Input: part model. Units: mm. Frame: model coordinates. A direction names the side the tool comes from. Give positions to 0.01 mm unless a question says otherwise; leave off trailing zeros. Write each loop counter-clockwise with the first axis right and the second up, starting at its lowest first coordinate (ties: lowest second). Pieces come first, ordered by that corner, then holes.
```python
from build123d import *

# Parameters (mm, degrees)
SKETCH1_W           = 85
SKETCH1_H           = 52.5
BOSS_EXTRUDE1_DEPTH = 27
SKETCH2_R           = 2.5
CUT_EXTRUDE1_DEPTH  = 104.490337713
SKETCH4_W           = 24.5
SKETCH4_H           = 12.7
CUT_EXTRUDE2_DEPTH  = 104.490337713
SKETCH5_W           = 25
SKETCH5_H           = 12.7
CUT_EXTRUDE3_DEPTH  = 94.477269964
SKETCH6_W           = 40.9
SKETCH6_H           = 28
CUT_EXTRUDE4_DEPTH  = 104.490337713
FILLET1_R           = 10
FILLET2_R           = 8
FILLET4_R           = 2
SKETCH7_R           = 2.75
CUT_EXTRUDE5_DEPTH  = 104.490337713
SKETCH8_W           = 6
SKETCH8_H           = 1.5
CUT_EXTRUDE6_DEPTH  = 2
CUT_EXTRUDE7_DEPTH  = 101.924427172
BOSS_EXTRUDE2_START = 17
BOSS_EXTRUDE2_DEPTH = 17
SKETCH11_R          = 2.75
CUT_EXTRUDE8_DEPTH  = 104.490337713
FILLET5_R           = 2


with BuildPart() as part:
    # Sketch1 → Boss-Extrude1 (new body)
    with BuildSketch(Plane(origin=(0, 0, 0), x_dir=(1, 0, 0), z_dir=(0, 1, 0))):
        with Locations((42.5, 26.25)):
            Rectangle(SKETCH1_W, SKETCH1_H)
    extrude(amount=BOSS_EXTRUDE1_DEPTH)

    # Sketch2 → Cut-Extrude1 (cut, through all)
    with BuildSketch(Plane(origin=(0, 27, 0), x_dir=(1, 0, 0), z_dir=(0, 1, 0))):
        with Locations(Location((5.5, 41.5, 0), (0, 0, 270))):
            Circle(SKETCH2_R)
        with Locations(Location((53.5, 41.5, 0), (0, 0, 270))):
            Circle(SKETCH2_R)
        with Locations(Location((53.5, 33.7, 0), (0, 0, 270))):
            Circle(SKETCH2_R)
        with Locations(Location((5.5, 33.7, 0), (0, 0, 270))):
            Circle(SKETCH2_R)
    extrude(amount=-CUT_EXTRUDE1_DEPTH, mode=Mode.SUBTRACT)

    # Sketch4 → Cut-Extrude2 (cut, through all)
    with BuildSketch(Plane.ZY):
        with Locations((-12.25, 20.65)):
            Rectangle(SKETCH4_W, SKETCH4_H)
    extrude(amount=-CUT_EXTRUDE2_DEPTH, mode=Mode.SUBTRACT)

    # Sketch5 → Cut-Extrude3 (cut, through all)
    with BuildSketch(Plane.XY.offset(-24.5)):
        with Locations((72.5, 20.65)):
            Rectangle(SKETCH5_W, SKETCH5_H)
    extrude(amount=-CUT_EXTRUDE3_DEPTH, mode=Mode.SUBTRACT)

    # Sketch6 → Cut-Extrude4 (cut, through all)
    with BuildSketch(Plane(origin=(0, 27, 0), x_dir=(1, 0, 0), z_dir=(0, 1, 0))):
        with Locations((29.5, 38.5)):
            Rectangle(SKETCH6_W, SKETCH6_H)
    extrude(amount=-CUT_EXTRUDE4_DEPTH, mode=Mode.SUBTRACT)

    # Fillet1
    # the kernel refuses this fillet: 10 mm, written as the material it takes off along each edge
    with BuildSketch(Plane(origin=(9.05, 51.886931812, -52.5), x_dir=(-1, 0, 0), z_dir=(0, -1, 0))) as fillet1_piece_1:
        with BuildLine():
            CenterArc((10, -9.954772725), FILLET1_R, 95.451319812, 84.548680188)
            Line((0, -9.954772725), (-0.2, -9.954772725))
            Line((-0.2, -9.954772725), (-0.2, 0))
            Line((-0.2, 0), (0, 0.2))
            ThreePointArc((0, 0.2), (4.525, 0.2), (9.031, 0.199095454))
            Line((9.031, 0.199095454), (9.05, 0))
        make_face()
    extrude(amount=76.773863623, mode=Mode.SUBTRACT)

    # Fillet2
    fillet2_edges = [part.edges().sort_by_distance(p)[0] for p in [
        (0, 20.65, -24.5),
        (60, 20.65, -52.5),
        (60, 20.65, -24.5),
    ]]
    fillet(fillet2_edges, radius=FILLET2_R)

    # Fillet4
    # the kernel refuses this fillet: 2 mm, written as the material it takes off along each edge
    with BuildSketch(Plane(origin=(9.05, 32.797158858, -24.5), x_dir=(0, 0, -1), z_dir=(0, -1, 0))) as fillet4_piece_1:
        with BuildLine():
            CenterArc((2.075685694, -2), FILLET4_R, 90, 99.110170153)
            Line((0.100914258, -2.316666667), (-0.096562885, -2.348333333))
            ThreePointArc((-0.096562885, -2.348333333), (-0.2, -1.05), (-0.2, 0))
            Line((-0.2, 0), (0, 0.2))
            Line((0, 0.2), (2.075685694, 0.2))
            Line((2.075685694, 0.2), (2.075685694, 0))
        make_face()
    extrude(amount=18.497158858, mode=Mode.SUBTRACT)
    with BuildSketch(Plane(origin=(49.95, 32, -24.5), x_dir=(0, 0, -1), z_dir=(0, -1, 0))) as fillet4_piece_2:
        with BuildLine():
            CenterArc((FILLET4_R, FILLET4_R), FILLET4_R, 180, 90)
            Line((0, FILLET4_R), (0, 0))
            Line((0, 0), (FILLET4_R, 0))
        make_face()
    extrude(amount=17.7, mode=Mode.SUBTRACT)
    with BuildSketch(Plane(origin=(49.95, 32, -52.5), x_dir=(0, 0, 1), z_dir=(0, -1, 0))) as fillet4_piece_3:
        with BuildLine():
            CenterArc((FILLET4_R, -FILLET4_R), FILLET4_R, 90, 90)
            Line((0, -FILLET4_R), (0, 0))
            Line((0, 0), (FILLET4_R, 0))
        make_face()
    extrude(amount=37, mode=Mode.SUBTRACT)
    with BuildSketch(Plane(origin=(85, -5, -52.5), x_dir=(0, 0, 1), z_dir=(0, 1, 0)), Plane(origin=(85, -5, 0), x_dir=(-1, 0, 0), z_dir=(0, 1, 0)), Plane(origin=(0, -5, 0), x_dir=(0, 0, -1), z_dir=(0, 1, 0))) as fillet4_piece_4:
        with BuildLine():
            CenterArc((FILLET4_R, -FILLET4_R), FILLET4_R, 90, 90)
            Line((0, -FILLET4_R), (0, 0))
            Line((0, 0), (FILLET4_R, 0))
        make_face()
    extrude(amount=24.3, mode=Mode.SUBTRACT)
    with BuildSketch(Plane(origin=(0, -7.039544043, -52.5), x_dir=(0.972186544788057, 0, 0.23420786095487744), z_dir=(0, 1, 0))) as fillet4_piece_5:
        with BuildLine():
            CenterArc((2.534235855, -1.980078713), FILLET4_R, 81.906386313, 111.638547186)
            Line((0.589862766, -2.448494435), (0, 0))
            ThreePointArc((0, 0), (1.407908809, 0.099606433), (2.815817617, 0))
        make_face()
    extrude(amount=41.079088086, mode=Mode.SUBTRACT)

    # Sketch7 → Cut-Extrude5 (cut, through all)
    with BuildSketch(Plane.XY):
        with Locations((70, 7.15)):
            Circle(SKETCH7_R)
        with Locations((20, 7.15)):
            Circle(SKETCH7_R)
    extrude(amount=-CUT_EXTRUDE5_DEPTH, mode=Mode.SUBTRACT)

    # Sketch8 → Cut-Extrude6 (cut)
    with BuildSketch(Plane(origin=(0, 27, 0), x_dir=(1, 0, 0), z_dir=(0, 1, 0))):
        with Locations((6.05, 37.6)):
            Rectangle(SKETCH8_W, SKETCH8_H)
        with Locations((52.95, 37.6)):
            Rectangle(SKETCH8_W, SKETCH8_H)
    extrude(amount=-CUT_EXTRUDE6_DEPTH, mode=Mode.SUBTRACT)

    # Sketch9 → Cut-Extrude7 (cut, through all)
    with BuildSketch(Plane(origin=(0, 14.3, 0), x_dir=(1, 0, 0), z_dir=(0, 1, 0))):
        with BuildLine():
            Line((85, 42.5), (60, 42.5))
            Line((60, 42.5), (60, 44.5))
            ThreePointArc((60, 44.5), (57.656854249, 50.156854249), (52, 52.5))
            Line((52, 52.5), (83, 52.5))
            Line((83, 52.5), (85, 52.5))
            Line((85, 52.5), (85, 42.5))
        make_face()
    extrude(amount=-CUT_EXTRUDE7_DEPTH, mode=Mode.SUBTRACT)

    # Sketch10 → Boss-Extrude2 (add)
    with BuildSketch(Plane.XZ.offset(BOSS_EXTRUDE2_START)):
        with BuildLine():
            Line((85, -42.5), (60, -42.5))
            Line((60, -42.5), (60, 0))
            Line((60, 0), (83, 0))
            ThreePointArc((83, 0), (84.414213562, -0.585786438), (85, -2))
            Line((85, -2), (85, -42.5))
        make_face()
    extrude(amount=-BOSS_EXTRUDE2_DEPTH)

    # Sketch11 → Cut-Extrude8 (cut, through all)
    with BuildSketch(Plane(origin=(85, 0, 0), x_dir=(0, 0, -1), z_dir=(1, 0, 0))):
        with Locations((30.5, -10)):
            Circle(SKETCH11_R)
        with Locations((12, -10)):
            Circle(SKETCH11_R)
    extrude(amount=-CUT_EXTRUDE8_DEPTH, mode=Mode.SUBTRACT)

    # Fillet5
    fillet5_edges = [part.edges().sort_by_distance(p)[0] for p in [
        (85, -1.35, -42.5),
        (60, -8.5, 0),
        (60, -8.5, -42.5),
    ]]
    fillet(fillet5_edges, radius=FILLET5_R)


solid = part.part
```
Q1. Section D-D, the plane y = 7.15. Return the cut outline in (x, z).
Q2. Mould query, pull axis X, two halves, no side actions, for faces 1 (the flat face through (55, 27, -39)), 2 (the cylindrical face through (4.54, 13.69, -39.19)), 3 (the flat face through (85, -2, -21)). Classes: +X half, -X half, draft (parallel to the pull), parting line (faces both ways), or undercut.
Q3. Access query for faces 4 (the cylindrical face through (50.55, 20.74, -25.07)), 5 (the cylindrical face through (60.57, -8.38, -0.6)), 6 (the cylindrical face through (60.6, -8.38, -41.93)). Directions: +Z, -Z, +X, -X, +Y, -Y. A direction counts if a zero-diameter tool reaches every point of the face in a straight line with its end or side. Return the directions, or none.
Q4. Material intervals for line 1 along X through (y, z) = (25, -33.5); line 2 along X through (y, z) = (13.5, -27.5); line 3 along X through (y, z) = (5.5, -33.7), sorted ascending.
Q5. Section A-A, the plane y = 21.5. Return the cut outline in (x, z), then the cut area to 3 significant figures.
Q6. Section B-B, the plane z = -12. Return the cut outline in (x, y), then the cut area to 3 significant figures.
Q7. Pin query (flat end, axial travel): pin 1 (0.6 mm diameter, centred on x = 5.5, y = 26.5, fed in from -Z); pin 2 (0.6 mm diameter, centred on x = 53.5, y = 26, fed in from -Z); pin 3 (0.8 mm diameter, centred on x = 54.5, z = -37.5, fed in from +Y); pin 4 (5 mm diameter, centred on y = -10, z = -12, fed in from +X). Return the tip coordinate at first contact, or that it passes through.
Q8. Section C-C, the plane x = 20. Return the cut outline in (y, z).
Solutions:
1. outline: (0, -49.98) arc R2 ccw to (2.74, -51.84) arc R10 ccw to (9.05, -42.55) - (9.05, -24.5) - (17.25, -24.5) - (17.25, 0) - (2, 0) arc R2 ccw to (0, -2) - close; (22.75, -24.5) - (49.95, -24.5) - (49.95, -50.5) arc R2 ccw to (51.95, -52.5) - (52, -52.5) arc R8 ccw to (60, -44.5) - (60, -42.5) - (67.25, -42.5) - (67.25, 0) - (22.75, 0) - close; (72.75, -42.5) - (83, -42.5) arc R2 ccw to (85, -40.5) - (85, -2) arc R2 ccw to (83, 0) - (72.75, 0) - close; hole circle Ø5 at (5.5, -41.5); hole circle Ø5 at (5.5, -33.7); hole circle Ø5 at (53.5, -41.5); hole circle Ø5 at (53.5, -33.7)
2. face 1: draft
2. face 2: undercut
2. face 3: +X half
3. face 4: +Z, +Y
3. face 5: +Z, -X, -Y
3. face 6: -Z, -X, -Y
4. line 1: x = 0 to 3.01, 7.99 to 9.05, 49.95 to 51.01, 55.99 to 60
4. line 2: x = 0 to 9.05, 49.95 to 85
4. line 3: x = 0 to 3, 8 to 9.05, 49.95 to 51, 56 to 67.8, 72.2 to 85
5. outline: (0, -49.98) arc R2 ccw to (2.74, -51.84) arc R10 ccw to (9.05, -42.55) - (9.05, -26.58) arc R2 ccw to (6.73, -24.6) arc R8 ccw to (0, -32.5) - close; (49.95, -50.5) arc R2 ccw to (51.95, -52.5) - (52, -52.5) arc R8 ccw to (60, -44.5) - (60, -32.5) arc R8 ccw to (52, -24.5) - (51.95, -24.5) arc R2 ccw to (49.95, -26.5) - close; hole circle Ø5 at (5.5, -41.5); hole circle Ø5 at (5.5, -33.7); hole circle Ø5 at (53.5, -41.5); hole circle Ø5 at (53.5, -33.7)
5. area: 390 mm2
6. outline: (0, 0) - (60, 0) - (60, -7.25) - (85, -7.25) - (85, 14.3) - (0, 14.3) - close; (60, -17) - (85, -17) - (85, -12.75) - (60, -12.75) - close; hole circle Ø5.5 at (20, 7.15); hole circle Ø5.5 at (70, 7.15)
6. area: 1,460 mm2
7. pin 1: stops at z = -50.43
7. pin 2: stops at z = -52.41
7. pin 3: stops at y = 25
7. pin 4: passes through
8. outline: (0, -24.5) - (4.4, -24.5) - (4.4, 0) - (0, 0) - close; (9.9, -24.5) - (14.3, -24.5) - (14.3, 0) - (9.9, 0) - close
